```python
from build123d import *

# Parameters (mm, degrees)
BOSS_EXTRUDE5_DEPTH  = 5
BOSS_EXTRUDE6_DEPTH  = 20.3
BOSS_EXTRUDE7_DEPTH  = 20
CUT_EXTRUDE1_DEPTH   = 90.151426067
CUT_EXTRUDE3_DEPTH   = 84.031866845
BOSS_EXTRUDE9_DEPTH  = 30
BOSS_EXTRUDE11_DEPTH = 20.3


with BuildPart() as part:
    # Sketch8 → Boss-Extrude5 (new body)
    with BuildSketch(Plane(origin=(0, 0, 0), x_dir=(1, 0, 0), z_dir=(0, 1, 0))):
        Polygon((-63.131930479, 24.805480282), (-52.701522962, -14.121330517), (0, -14.121330517), (0, 41.721630071), align=None)
    boss_extrude5 = extrude(amount=BOSS_EXTRUDE5_DEPTH)

    # Sketch9 → Boss-Extrude6 (add)
    with BuildSketch(Plane(origin=(0, 5, 0), x_dir=(1, 0, 0), z_dir=(0, 1, 0))):
        Polygon((-63.131930479, 24.805480282), (-57.955549577, 5.486963756), (0, 21.016106462), (0, 41.721630071), align=None)
    boss_extrude6 = extrude(amount=BOSS_EXTRUDE6_DEPTH)

    # Sketch10 → Boss-Extrude7 (add)
    with BuildSketch(Plane(origin=(0, 25.3, 0), x_dir=(1, 0, 0), z_dir=(0, 1, 0))):
        Polygon((0, 41.721630071), (0, -14.121330517), (-52.701522962, -14.121330517), (-63.131930479, 24.805480282), align=None)
    boss_extrude7 = extrude(amount=BOSS_EXTRUDE7_DEPTH)

    # Sketch19 → Cut-Extrude1 (cut, through all)
    with BuildSketch(Plane(origin=(-52.701522962, 0, 14.121330517), x_dir=(0.25881904510251774, 0, 0.9659258262890692), z_dir=(-0.9659258262890692, 0, 0.25881904510251774))):
        Polygon((-32.255495471, 0), (-20.117397053, 45.3), (-40.3, 45.3), (-40.3, 0), align=None)
    cut_extrude1 = extrude(amount=-CUT_EXTRUDE1_DEPTH, mode=Mode.SUBTRACT)

    # Sketch22 → Cut-Extrude3 (cut, through all)
    with BuildSketch(Plane(origin=(0, 0, 0), x_dir=(0, 0, -1), z_dir=(1, 0, 0))):
        Polygon((-14.121330517, 30.3), (22.193593674, 40.37381141), (20.827061981, 45.3), (-14.121330517, 45.3), align=None)
    cut_extrude3 = extrude(amount=-CUT_EXTRUDE3_DEPTH, mode=Mode.SUBTRACT)

    # Sketch23 → Boss-Extrude9 (add)
    with BuildSketch(Plane(origin=(0, 31.772345951, 8.813693772), x_dir=(1, 0, 0), z_dir=(0, 0.9636113749942826, 0.26730716036355656))):
        Polygon((-10.15, -5.508067758), (-15.15, -5.508067758), (-15.15, 19.791932242), (0, 19.791932242), (0, 14.791932242), (-10.15, 14.791932242), align=None)
    boss_extrude9 = extrude(amount=BOSS_EXTRUDE9_DEPTH)

    # Sketch24 → Boss-Extrude11 (add)
    with BuildSketch(Plane(origin=(0, 5, 0), x_dir=(1, 0, 0), z_dir=(0, 1, 0))):
        Polygon((-2.5, -14.121330517), (-11.116891, 18.037344497), (0, 21.016106462), (0, -14.121330517), align=None)
    boss_extrude11 = extrude(amount=BOSS_EXTRUDE11_DEPTH)

    # Mirror1: Boss-Extrude5, Boss-Extrude6, Boss-Extrude7, Cut-Extrude1, Cut-Extrude3, Boss-Extrude9, Boss-Extrude11 across plane
    add(boss_extrude5.mirror(Plane(origin=(0, 5, -41.721630071), x_dir=(0, 0, 1), z_dir=(-1, 0, 0))))
    add(boss_extrude6.mirror(Plane(origin=(0, 5, -41.721630071), x_dir=(0, 0, 1), z_dir=(-1, 0, 0))))
    add(boss_extrude7.mirror(Plane(origin=(0, 5, -41.721630071), x_dir=(0, 0, 1), z_dir=(-1, 0, 0))))
    add(cut_extrude1.mirror(Plane(origin=(0, 5, -41.721630071), x_dir=(0, 0, 1), z_dir=(-1, 0, 0))), mode=Mode.SUBTRACT)
    add(cut_extrude3.mirror(Plane(origin=(0, 5, -41.721630071), x_dir=(0, 0, 1), z_dir=(-1, 0, 0))), mode=Mode.SUBTRACT)
    add(boss_extrude9.mirror(Plane(origin=(0, 5, -41.721630071), x_dir=(0, 0, 1), z_dir=(-1, 0, 0))))
    add(boss_extrude11.mirror(Plane(origin=(0, 5, -41.721630071), x_dir=(0, 0, 1), z_dir=(-1, 0, 0))))


solid = part.part
```
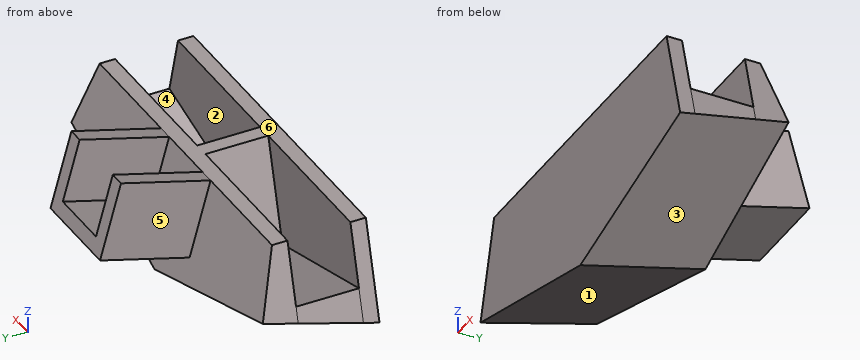
Geometry check sheet. Reference: the model listing, model coordinates, mm. Face numbers are marked on the shaded views. A direction names the side the tool comes from. Give positions to 0.01 mm unless a question says otherwise; leave off trailing zeros. Order: outer loops, then holes, each group sorted by start corner. A loop starts at its lowest first (then second) coordinate and runs counter-clockwise, first axis right, second up. Notation, with made-up numbers: (13, 1.25) -> (37, 1.25) arc R14 cw to (37, 21.25) -> close; hole circle Ø6 at (80, -8). An arc over 180 degrees is marked (long way). Write each question's results on one line, items separated by ' | '. Start each with the question number.
(1) Sectioned sample at C-C (z = 17.5). Enter the section's corners in (x, y).
(2) Access from +Z, -Z, +X, -X, +Y, -Y to the whole of each face (thin tool, end or side, straight path). Record for the marked faces 4, 5 and 6.
(3) Gauge pin test, flat ends, axial feed: P1, Ø5, axis at y = 15, z = 0, coming from the +X side; P2, Ø14, axis at y = 40.5, z = 9.5, coming from the -X side; P3, Ø14, axis at y = 44, z = 14.5, coming from the +X side; P4, Ø12, axis at x = -1.5, z = -5.5, coming from the -Y side. Record the tip position at first contact, or that the pin passes through.
(4) Sectioned sample at D-D (y = 45). Enter the section's corners in (x, z), plus the area to 3 significant figures.
(5) Sectioned sample at A-A (z = -4). Enter the section's corners in (x, y), plus the area to 3 significant figures.
(6) Mould release check, pull along X, two halves, no side actions. Record for the marked faces 1, 2 and 3: pulls with the +X half, pulls with the -X half, needs draft (parallel to the pull), parting line crosses it, or undercut.
(7) Scan lines: line 1 (Y direction, x = -51, z = -6); line 2 (Y direction, x = 17.5, z = -13); line 3 (Z direction, x = 17, y = 8). Record each from-to range of solid material in increasing order.
(8) Sectioned sample at B-B (x = -36). Enter the section's corners in (y, z), plus the area to 3 significant figures.
Answer below:
1) outline: (-15.15, 42.48) -> (-10.15, 42.48) -> (-10.15, 60.5) -> (-15.15, 60.5) -> close; (10.15, 42.48) -> (15.15, 42.48) -> (15.15, 60.5) -> (10.15, 60.5) -> close
2) face 4: +Z | face 5: +Z, -X, +Y | face 6: +Z, +X, -X, -Y
3) P1: x = 6.95 | P2: x = -15.15 | P3: x = 15.15 | P4: y = 0
4) outline: (-15.15, -8.06) -> (15.15, -8.06) -> (15.15, 18.2) -> (10.15, 18.2) -> (10.15, -2.87) -> (-10.15, -2.87) -> (-10.15, 18.2) -> (-15.15, 18.2) -> close | area: 368 mm2
5) outline: (-57.56, 0) -> (57.56, 0) -> (57.56, 5) -> (7.36, 5) -> (7.36, 25.3) -> (57.56, 25.3) -> (57.56, 35.33) -> (15.15, 35.33) -> (15.15, 59.62) -> (-15.15, 59.62) -> (-15.15, 35.33) -> (-57.56, 35.33) -> (-57.56, 25.3) -> (-7.36, 25.3) -> (-7.36, 5) -> (-57.56, 5) -> close; hole (-10.15, 35.33) -> (10.15, 35.33) -> (10.15, 40.92) -> (-10.15, 40.92) -> close | area: 2,650 mm2
6) face 1: pulls with the -X half | face 2: undercut | face 3: pulls with the +X half
7) line 1: 0 to 5, 25.3 to 35.88 | line 2: 0 to 5, 25.3 to 37.82 | line 3: -26.62 to -16.46
8) outline: (0, -23.75) -> (37.89, -13.24) -> (30.3, 14.12) -> (25.3, 14.12) -> (25.3, -11.37) -> (5, -11.37) -> (5, 14.12) -> (0, 14.12) -> close | area: 614 mm2
